from build123d import *

# Parameters (mm, degrees)
F1_DEPTH = 1676.4
F2_T     = -3.175
F3_DEPTH = 25.4
F4_DEPTH = 25.4
F6_DEPTH = 3.175


with BuildPart() as f1:
    # F0 (on Front) → F1 (new body)
    with BuildSketch(Plane.XZ):
        Polygon((-22.225, 0), (0, 0), (22.225, 0), (44.45, 101.6), (-44.45, 101.6), align=None)
    extrude(amount=F1_DEPTH)

    # F2
    f2_openings = [f1.faces().sort_by_distance(p)[0] for p in [
        (0, -838.2, 101.6),
    ]]
    offset(amount=F2_T, openings=f2_openings)

    # F3 (cut): a face of the model
    f3_faces = [f1.faces().sort_by_distance(p)[0] for p in [
        (0, -1673.225, 58.1899151132),
    ]]
    extrude(f3_faces, amount=-F3_DEPTH, mode=Mode.SUBTRACT)

    # F4 (cut): a face of the model
    f4_faces = [f1.faces().sort_by_distance(p)[0] for p in [
        (0, -3.175, 58.1899151132),
    ]]
    extrude(f4_faces, amount=-F4_DEPTH, mode=Mode.SUBTRACT)

    # F5 (on face) → F6 (join)
    with BuildSketch(Plane.XZ.offset(1676.4)):
        Polygon((69.85, 101.6), (44.45, 101.6), (22.225, 0), (-22.225, 0), (-44.45, 101.6), (-69.85, 101.6), (-69.85, -50.8), (69.85, -50.8), align=None)
    extrude(amount=-F6_DEPTH)


solid = f1.part
Design review of the part built by this model. Coordinates are the model's own, in mm. A direction names the side the tool comes from. Give positions to 0.01 mm unless a question says otherwise; leave off trailing zeros. Loops run counter-clockwise (first coordinate to the right, second up) from the corner with the lowest first, then second, coordinate; pieces in that order, holes last. Notation, with made-up numbers: (77, 59) - (120, 59) arc R20 ccw to (120, 70) - close; hole circle Ø3 at (19.25, 69.5). An arc over 180 degrees is marked (long way). Write item = value, one per line.
1) Take a section at B-B on y = -318. State the section outline as (x, z) points (3 decimals).
Result sheet:
outline = (-44.45, 101.6) - (-22.225, 0) - (22.225, 0) - (44.45, 101.6) - (41.2, 101.6) - (19.669, 3.175) - (-19.669, 3.175) - (-41.2, 101.6) - close
2) Tool access review of faces 1 (the face through (30.284, -849.935, 51.699)), 2 (the face through (33.182, -824.9, 50.089)), 3 (the face through (-33.493, -824.9, 51.511)), 4 (the face through (0, -825, 0)): name each direction out of +Z, -Z, +X, -X, +Y, -Y from which nothing blocks a thin tool from reaching the whole face with its end or side.
Result sheet:
face_1 = +Z, +Y, -Y
face_2 = -Z, +X, +Y
face_3 = -Z, -X, +Y
face_4 = -Z, +X, -X, +Y
3) Clearance check with flat-ended pins moving along their axes: pin 1 Ø3 at (y, z) = (-514.5, 21.5) entering from +X; pin 2 Ø5 at (y, z) = (-248.5, 78) entering from -X; pin 3 Ø6 at (y, z) = (-1030, 7) entering from -X. State where each tip first meets the part, or that it passes through.
Result sheet:
pin_1 = 27.26
pin_2 = -39.83
pin_3 = -24.41
4) Take a section at C-C on x = -5.5. State the section outline as (y, z) points (3 decimals), and give its area (3 significant figures).
Result sheet:
outline = (-1676.4, -50.8) - (-1673.225, -50.8) - (-1673.225, 0) - (0, 0) - (0, 3.175) - (-1676.4, 3.175) - close
area = 5,480 mm2
5) Take a section at A-A on z = 71.5. State the section outline as (x, y) points (3 decimals).
Result sheet:
outline = (-69.85, -1676.4) - (-34.616, -1676.4) - (-34.616, 0) - (-37.866, 0) - (-37.866, -1673.225) - (-69.85, -1673.225) - close; (34.616, -1676.4) - (69.85, -1676.4) - (69.85, -1673.225) - (37.866, -1673.225) - (37.866, 0) - (34.616, 0) - close
6) Take a section at D-D on z = -24. State the section outline as (x, y) points (3 decimals), and give its area (3 significant figures).
Result sheet:
outline = (-69.85, -1676.4) - (69.85, -1676.4) - (69.85, -1673.225) - (-69.85, -1673.225) - close
area = 444 mm2
7) To check wall thickness, follow line 1 (Z direction, x = 11, y = -796.5) (3 decimals); line 2 (Y direction, x = 56, z = 36) (3 decimals); line 3 (X direction, y = -980.5, z = 69). State the ranges of each line that lie inside material, in increasing order.
Result sheet:
line_1 = 0 to 3.175
line_2 = -1676.4 to -1673.225
line_3 = -37.32 to -34.07, 34.07 to 37.32
